Read the model definition and answer for the solid it produces. Units are mm, in the model's axes. A direction names the side the tool comes from. Coordinates: 2 decimals unless noted, no trailing zeros. Order: outer loops, then holes, each group sorted by start corner. A loop starts at its lowest first (then second) coordinate and runs counter-clockwise, first axis right, second up. Notation, with made-up numbers: (-36, -25) - (12, -25) arc R26 ccw to (12, -8) - close; hole circle Ø6 at (7.5, 51). An arc over 180 degrees is marked (long way). Use one line per item in the form item = value.
```python
from build123d import *

# Parameters (mm, degrees)
BOSS_EXTRUDE1_DEPTH = 76.2
FILLET1_R           = 7.874
SKETCH3_R           = 12.7
SKETCH3_R_2         = 10
CUT_EXTRUDE1_DEPTH  = 15.748


with BuildPart() as part:
    # Sketch1 → Boss-Extrude1 (new body, symmetric)
    with BuildSketch(Plane.XY):
        Polygon((-136.652, 127), (-152.4, 127), (-152.4, 0), (152.4, 0), (152.4, 127), (136.652, 127), (136.652, 8.89), (-136.652, 8.89), align=None)
    extrude(amount=BOSS_EXTRUDE1_DEPTH, both=True)

    # Fillet1
    fillet1_edges = [part.edges().sort_by_distance(p)[0] for p in [
        (-136.652, 8.89, 0),
        (136.652, 8.89, 0),
        (136.652, 127, 0),
        (-136.652, 127, 0),
    ]]
    fillet(fillet1_edges, radius=FILLET1_R)

    # Sketch3 → Cut-Extrude1 (cut)
    with BuildSketch(Plane(origin=(152.4, 0, 0), x_dir=(0, 0, -1), z_dir=(1, 0, 0))):
        with Locations((50.506866673, 50.8)):
            Circle(SKETCH3_R)
        with Locations((-54.493133327, 50.8)):
            Circle(SKETCH3_R)
        with Locations((-1.993133327, 50.8)):
            Circle(SKETCH3_R_2)
    extrude(amount=-CUT_EXTRUDE1_DEPTH, mode=Mode.SUBTRACT)


solid = part.part
```
(1) Section A-A, the plane y = 50.8 is taken. Write down the section's boundary in (x, z), then the cut area to 3 significant figures.
Answer list:
outline = (-152.4, -76.2) - (-136.65, -76.2) - (-136.65, 76.2) - (-152.4, 76.2) - close; (136.65, -76.2) - (152.4, -76.2) - (152.4, -63.21) - (136.65, -63.21) - close; (136.65, -37.81) - (152.4, -37.81) - (152.4, -8.01) - (136.65, -8.01) - close; (136.65, 11.99) - (152.4, 11.99) - (152.4, 41.79) - (136.65, 41.79) - close; (136.65, 67.19) - (152.4, 67.19) - (152.4, 76.2) - (136.65, 76.2) - close
area = 3,690 mm2
(2) Section D-D, the plane x = 20.5 is taken. Write down the section's boundary in (y, z).
Answer list:
outline = (0, -76.2) - (8.89, -76.2) - (8.89, 76.2) - (0, 76.2) - close
(3) The mould has two halves that part along Z. Classify faces 4 (the flat face through (-1, 7, -76.2)), 5 (the flat face through (149, 127, 1)), 6 (the flat face through (-1, 7, 76.2)), 7 (the cylindrical face through (144.64, 45.94, 42.76)): +Z half, -Z half, draft (parallel to the pull), parting line (faces both ways), or undercut.
Answer list:
face_4 = -Z half
face_5 = draft
face_6 = +Z half
face_7 = undercut
(4) Given pin 1 Ø1 at (x, z) = (-80, 39.5) entering from -Y; pin 2 Ø12 at (y, z) = (50.8, 1.99) entering from +X; pin 3 Ø1.5 at (x, z) = (-22.5, 17) entering from +Y, each flat-ended and moving along its own axis, determine where each tip first touches the part or whether it passes through.
Answer list:
pin_1 = 0
pin_2 = -136.65
pin_3 = 8.89
(5) Straight lines are drawn through the part: L1, parallel to Z at x = 147, y = 50; L2, parallel to X at y = 34, z = 38; L3, parallel to Y at x = -94, z = 17. For each, find the intervals that lie inside material, in ascending order.
Answer list:
L1 = -76.2 to -63.18, -37.83 to -7.97, 11.96 to 41.82, 67.17 to 76.2
L2 = -152.4 to -136.65, 136.65 to 152.4
L3 = 0 to 8.89
(6) Section C-C, the plane z = 21 is taken. Write down the section's boundary in (x, y), then the cut area to 3 significant figures.
Answer list:
outline = (-152.4, 0) - (152.4, 0) - (152.4, 127) - (144.53, 127) arc R7.87 ccw to (136.65, 119.13) - (136.65, 16.76) arc R7.87 cw to (128.78, 8.89) - (-128.78, 8.89) arc R7.87 cw to (-136.65, 16.76) - (-136.65, 119.13) arc R7.87 ccw to (-144.53, 127) - (-152.4, 127) - close
area = 6,430 mm2
(7) Section B-B, the plane z = -41 is taken. Write down the section's boundary in (x, y), then the cut area to 3 significant figures.
Answer list:
outline = (-152.4, 0) - (152.4, 0) - (152.4, 42.38) - (136.65, 42.38) - (136.65, 16.76) arc R7.87 cw to (128.78, 8.89) - (-128.78, 8.89) arc R7.87 cw to (-136.65, 16.76) - (-136.65, 119.13) arc R7.87 ccw to (-144.53, 127) - (-152.4, 127) - close; (136.65, 59.22) - (152.4, 59.22) - (152.4, 127) - (144.53, 127) arc R7.87 ccw to (136.65, 119.13) - close
area = 6,160 mm2
(8) Which of the six approach directions +Z, -Z, +X, -X, +Y, -Y give full straight-line access (tool end or side, diameter ignored) to faces 1 (the flat face through (-136.652, 67, 1)), 2 (the cylindrical face through (144.636, 60.715, 3.295)), 3 (the flat face through (-148, 127, 1))?
Answer list:
face_1 = +Z, -Z, +Y
face_2 = +X
face_3 = +Z, -Z, +X, -X, +Y
